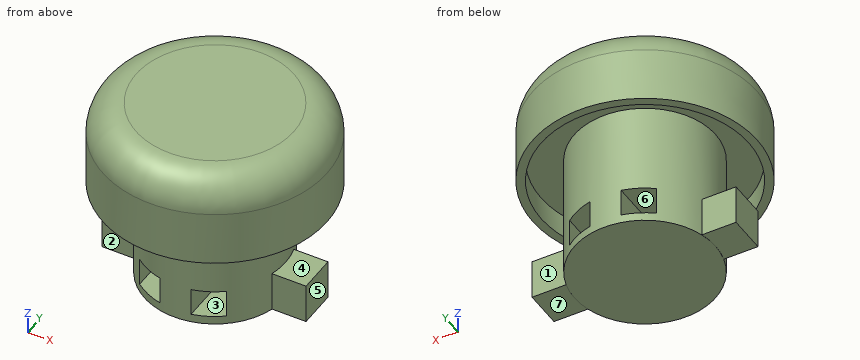
```python
from build123d import *

# Parameters (mm, degrees)
SKETCH1_R               = 42.5
BOSS_EXTRUDE1_DEPTH     = 76
SKETCH2_R               = 67.5
BOSS_EXTRUDE2_DEPTH     = 39
FILLET1_R               = 20
BOSS_EXTRUDE3_START     = 14
SKETCH3_R               = 67.5
SKETCH3_R_2             = 62.5
BOSS_EXTRUDE3_DEPTH     = 14
SKETCH4_W               = 123
SKETCH4_H               = 24.049182643
BOSS_EXTRUDE4_DEPTH     = 11.5
CUT_EXTRUDE1_DEPTH      = 150.457351776
CUT_EXTRUDE1_DEPTH_BACK = 150.457351776
SKETCH5_W               = 16.750654132
SKETCH5_H               = 16.750654132


with BuildPart() as part:
    # Sketch1 → Boss-Extrude1 (new body)
    with BuildSketch(Plane.XY):
        Circle(SKETCH1_R)
    extrude(amount=BOSS_EXTRUDE1_DEPTH)

    # Sketch2 → Boss-Extrude2 (add)
    with BuildSketch(Plane.XY.offset(76)):
        Circle(SKETCH2_R)
    extrude(amount=BOSS_EXTRUDE2_DEPTH)

    # Fillet1
    fillet1_edges = [part.edges().sort_by_distance(p)[0] for p in [
        (-67.5, 0, 115),
    ]]
    fillet(fillet1_edges, radius=FILLET1_R)

    # Sketch3 → Boss-Extrude3 (add)
    with BuildSketch(Plane(origin=(0, 0, 76), x_dir=(-1, 0, 0), z_dir=(0, 0, -1)).offset(BOSS_EXTRUDE3_START)):
        Circle(SKETCH3_R)
        Circle(SKETCH3_R_2, mode=Mode.SUBTRACT)
    extrude(amount=-BOSS_EXTRUDE3_DEPTH)

    # Sketch4 → Boss-Extrude4 (add, symmetric)
    with BuildSketch(Plane(origin=(0, 0, 0), x_dir=(1, 0, 0), z_dir=(0, 1, 0))):
        with Locations((0, -12.155455807)):
            Rectangle(SKETCH4_W, SKETCH4_H)
    extrude(amount=BOSS_EXTRUDE4_DEPTH, both=True)

    # Sketch5 → Cut-Extrude1 (cut, two sides: drawn at the far end of the back side and taken through both)
    with BuildSketch(Plane(origin=(0, 0, 0), x_dir=(1, 0, 0), z_dir=(0, 1, 0)).offset(-CUT_EXTRUDE1_DEPTH_BACK)):
        with Locations((-17.797570015, -13.464100661)):
            Rectangle(SKETCH5_W, SKETCH5_H)
        with Locations((17.797570015, -13.464100661)):
            Rectangle(SKETCH5_W, SKETCH5_H)
    extrude(amount=CUT_EXTRUDE1_DEPTH + CUT_EXTRUDE1_DEPTH_BACK, mode=Mode.SUBTRACT)


solid = part.part
```
Build history of the part. All positions in model axes, mm. Face numbers are marked on the shaded views. A direction names the side the tool comes from. Round coordinates to 2 decimals unless told otherwise and drop trailing zeros. Loops run counter-clockwise (first coordinate to the right, second up) from the corner with the lowest first, then second, coordinate; pieces in that order, holes last.
Item 1: Drill centre lines: line 1 along Y through (x, z) = (0, 68); line 2 along Z through (x, y) = (24, 29); line 3 along X through (y, z) = (-17.5, 19). Where is each one in solid material? Low to high.
Item 2: Which spindle directions (+Z, -Z, +X, -X, +Y, -Y) get a long thin tool onto all of the face, cutting with end or side? Do the marked faces 1, 2 and 3. Say none if no direction does.
Item 3: Two-plate mould, pull along Z, no slides. Class the marked faces 4, 5, 6 and 7: released by +Z, released by -Z, zero draft, split by the parting line, or undercut.
Item 4: Saw through at B-B (x = 0). List the corners of the cut face in (y, z).
Item 5: Pin check, flat tips, straight feed: P1, Ø6, axis at y = -3, z = 46, coming from the -X side; P2, Ø3, axis at y = -26.5, z = 59, coming from the +X side; P3, Ø6, axis at x = 50, z = 11.5, coming from the +Y side; P4, Ø10.5, axis at x = 50, y = 4, coming from the +Z side. Stop position of each tip, or through.
Item 6: Saw through at A-A (y = 0). State how many separate pieces and enclosed holes the cut face has, then the cut area to 3 significant figures.
Item 7: Saw through at C-C (z = 85.5). List the corners of the cut face in (x, y), then the cut area to 3 significant figures.
Worked answers:
1. line 1: y = -67.5 to -62.5, -42.5 to 42.5, 62.5 to 67.5
1. line 2: z = 0 to 5.09, 21.84 to 115
1. line 3: x = -38.73 to -26.17, -9.42 to 9.42, 26.17 to 38.73
2. face 1: -Z, +X, +Y
2. face 2: -Z, -X, -Y
2. face 3: +Y, -Y
3. face 4: undercut
3. face 5: zero draft
3. face 6: undercut
3. face 7: released by -Z
4. outline: (-67.5, 62) - (-62.5, 62) - (-62.5, 76) - (-42.5, 76) - (-42.5, 0) - (42.5, 0) - (42.5, 76) - (62.5, 76) - (62.5, 62) - (67.5, 62) - (67.5, 95) arc R20 ccw to (47.5, 115) - (-47.5, 115) arc R20 ccw to (-67.5, 95) - close
5. P1: stops at x = -42.5
5. P2: stops at x = 34.37
5. P3: stops at y = 11.5
5. P4: stops at z = 115
6. separate pieces: 1
6. enclosed holes: 2
6. area: 12,000 mm2
7. outline: circle Ø135 at (0, 0)
7. area: 14,300 mm2
